```python
from build123d import *

# Parameters (mm, degrees)
SKETCH3_W          = 16
SKETCH3_H          = 1.5
CHAMFER1_SIZE      = 0.45
CUT_EXTRUDE1_DEPTH = 1.19


with BuildPart() as part:
    # Sketch3 → Revolve1 (revolve)
    with BuildSketch(Plane(origin=(0, 0, 0), x_dir=(0, 0, -1), z_dir=(1, 0, 0))):
        with Locations((0, 0.75)):
            Rectangle(SKETCH3_W, SKETCH3_H)
    revolve(axis=Axis((0, 0, -8), (0, 0, 1)))

    # Chamfer1
    chamfer1_edges = [part.edges().sort_by_distance(p)[0] for p in [
        (0, -1.5, -8),
    ]]
    chamfer(chamfer1_edges, length=CHAMFER1_SIZE)

    # Sketch6 → Revolve2 (revolve)
    with BuildSketch(Plane(origin=(0, 0, 0), x_dir=(0, 0, -1), z_dir=(1, 0, 0))):
        Polygon((-8, 3), (-7.8, 3), (-6.3, 1.5), (-6.3, 0), (-8, 0), align=None)
    revolve(axis=Axis((0, 0, -8), (0, 0, 1)))

    # Sketch8 → Cut-Extrude1 (cut)
    with BuildSketch(Plane.XY.offset(8)):
        Polygon((0, 1.154700538), (-1, 0.577350269), (-1, -0.577350269), (0, -1.154700538), (1, -0.577350269), (1, 0.577350269), align=None)
    extrude(amount=-CUT_EXTRUDE1_DEPTH, mode=Mode.SUBTRACT)

    # Cut-Extrude2 cone 1 section (through the dimple's axis) → Cut-Extrude2 (revolve, cut)
    with BuildSketch(Plane(origin=(0, 0, 8), x_dir=(0, -1, 0), z_dir=(1, 0, 0))):
        Polygon((0, 0), (1.154700538, 0), (0, 1.154700538), align=None)
    revolve(axis=Axis((0, 0, 8), (0, 0, -1)), mode=Mode.SUBTRACT)


solid = part.part
```
Work out the finished part from the listing and answer in its coordinate system (mm). A direction names the side the tool comes from. Give positions to 0.01 mm unless a question says otherwise; leave off trailing zeros. Order: outer loops, then holes, each group sorted by start corner. A loop starts at its lowest first (then second) coordinate and runs counter-clockwise, first axis right, second up. Notation, with made-up numbers: (67.5, 88.5) -> (117.5, 88.5) arc R16 ccw to (117.5, 112.5) -> close; hole circle Ø8 at (15.5, 80). An arc over 180 degrees is marked (long way). Answer as CSV lines item,"result". Start each with the question number.
(1) Section B-B, the plane z = -5.5 is taken. Write down the section's boundary in (x, y).
(2) Each of these flat-tipped pins is pushed along its axis until it touches: pin 1 Ø1 at (y, z) = (-2.5, -6) entering from +X; pin 2 Ø1.6 at (x, y) = (0, 0) entering from +Z. Where does it stop, or does it pass through?
(3) Section A-A, the plane y = 0 is taken. Write down the section's boundary in (x, z), plus the area to 3 significant figures.
(4) Which of the six approach directions +Z, -Z, +X, -X, +Y, -Y give full straight-line access (tool end or side, diameter ignored) to faces 5 (the flat face through (-0.51, -0.86, 7.41)), 6 (the flat face through (0, 0, -8))?
(5) Consider line 1 along Y through (x, z) = (-0.4, 7.25); line 2 along Y through (x, z) = (-1.3, -1.5); line 3 along X through (y, z) = (0.9, -4.75). Determine where each line is inside the solid, lowest interval first.
(6) For a pull along Y with two mould halves and no side action, classify faces 1 (the flat face through (1, -1, 8)), 2 (the flat face through (0, 0, 6.81)), 3 (the cylindrical face through (-0.07, -1.5, -0.72)), 4 (the flat face through (0.51, 0.86, 7.41)) as released by +Y, released by -Y, zero draft, split by the parting line, or undercut.
Entries:
1,outline,"circle Ø3 at (0, 0)"
2,pin 1,"through"
2,pin 2,"z = 6.81"
3,outline,"(-3, 7.8) -> (-1.5, 6.3) -> (-1.5, -7.55) -> (-1.05, -8) -> (1.05, -8) -> (1.5, -7.55) -> (1.5, 6.3) -> (3, 7.8) -> (3, 8) -> (1.15, 8) -> (1, 7.85) -> (1, 6.81) -> (-1, 6.81) -> (-1, 7.85) -> (-1.15, 8) -> (-3, 8) -> close"
3,area,"48.2 mm²"
4,face 5,"+Z"
4,face 6,"-Z, +X, -X, +Y, -Y"
5,line 1,"-2.42 to -0.92, 0.92 to 2.42"
5,line 2,"-0.75 to 0.75"
5,line 3,"-1.2 to 1.2"
6,face 1,"zero draft"
6,face 2,"undercut"
6,face 3,"split by the parting line"
6,face 4,"undercut"
